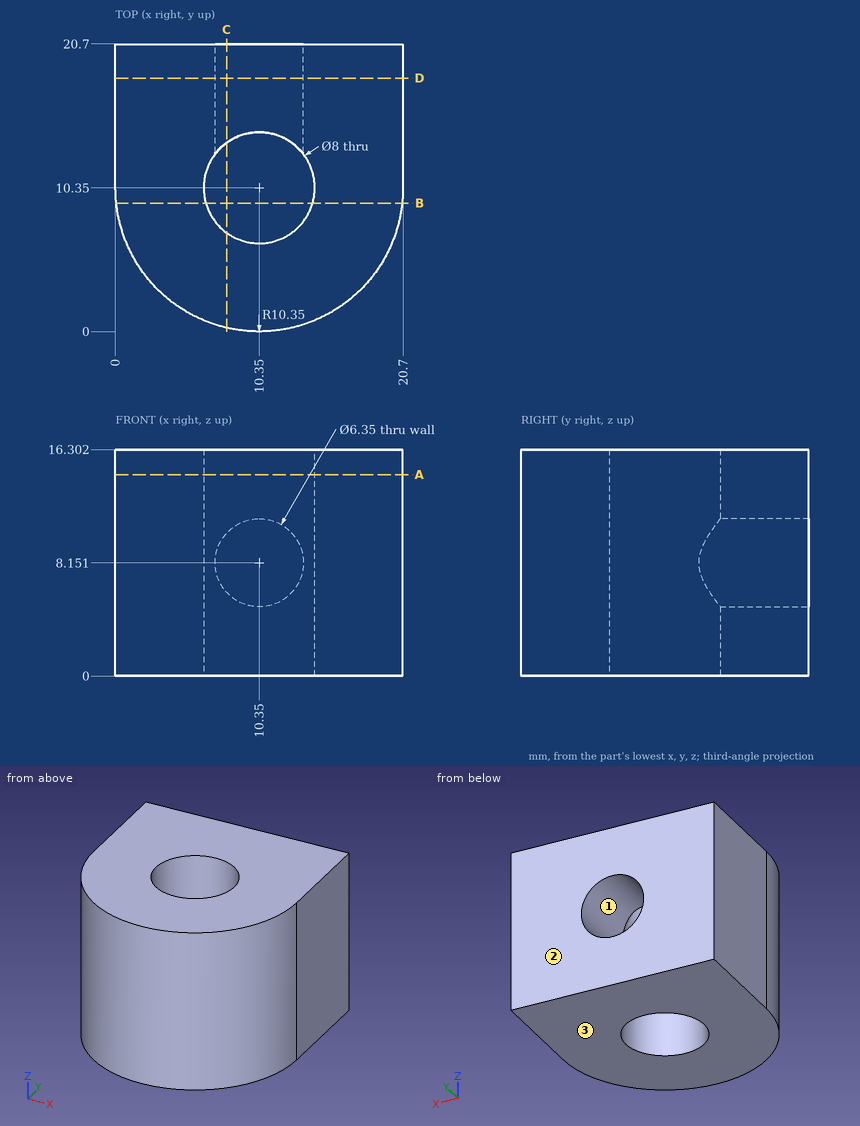
Drawing for the job (mm, zero at the part's lowest x, y, z). Round coordinates to 2 decimals unless told otherwise and drop trailing zeros. Write each loop counter-clockwise with the first axis right and the second up, starting at its lowest first coordinate (ties: lowest second). Pieces come first, ordered by that corner, then holes.
Item 1: Drill centre lines: L1, parallel to X at y = 10.5, z = 11.75; L2, parallel to Y at x = 13, z = 13 (3 decimals); L3, parallel to X at y = 7.25, z = 11.75 (3 decimals). Where is each one in solid material? Low to high.
Filled in:
L1: x = 0 to 6.35, 14.35 to 20.7
L2: y = 0.345 to 7.354, 13.346 to 20.7
L3: x = 0.475 to 7.822, 12.878 to 20.225
Item 2: Band-saw the part on B-B on y = 9.25. Write the cut outline in (x, z), then the cut area to 3 significant figures.
Filled in:
outline: (0.06, 0) - (6.5, 0) - (6.5, 16.3) - (0.06, 16.3) - close; (14.2, 0) - (20.64, 0) - (20.64, 16.3) - (14.2, 16.3) - close
area: 210 mm2
Item 3: Band-saw the part on A-A on z = 14.5. Write the cut outline in (x, y), then the cut area to 3 significant figures.
Filled in:
outline: (0, 10.35) arc R10.35 ccw to (20.7, 10.35) - (20.7, 20.7) - (0, 20.7) - close; hole circle Ø8 at (10.35, 10.35)
area: 332 mm2
Item 4: Band-saw the part on D-D on y = 18.25. Write the cut outline in (x, z) (3 decimals), then the cut area to 3 significant figures.
Filled in:
outline: (0, 0) - (20.7, 0) - (20.7, 16.302) - (0, 16.302) - close; hole circle Ø6.35 at (10.35, 8.151)
area: 306 mm2
Item 5: Drop flat-ended pins along their axis: pin 1 Ø5.5 at (x, z) = (10.35, 8.15) entering from +Y; pin 2 Ø1.5 at (x, z) = (14, 13.5) entering from -Y; pin 3 Ø1 at (y, z) = (9, 13.5) entering from -X (3 decimals); pin 4 Ø6.5 at (x, y) = (10.35, 10.35) entering from -Z (3 decimals). Give the stop position or say it passes through.
Filled in:
pin 1: stops at y = 7.45
pin 2: stops at y = 0.41
pin 3: stops at x = 0.035
pin 4: passes through
Item 6: Mould opens along Z. For the marked faces 1, 2 and 3 say: released by +Z, released by -Z, zero draft, split by the parting line, or undercut.
Filled in:
face 1: undercut
face 2: zero draft
face 3: released by -Z
Item 7: Band-saw the part on C-C on x = 8. Write the cut outline in (y, z).
Filled in:
outline: (0.27, 0) - (7.11, 0) - (7.11, 16.3) - (0.27, 16.3) - close; (13.59, 0) - (20.7, 0) - (20.7, 6.02) - (13.59, 6.02) - close; (13.59, 10.29) - (20.7, 10.29) - (20.7, 16.3) - (13.59, 16.3) - close
